Could you check a few things on this model? Use its own coordinates, in mm. A direction names the side the tool comes from. Give positions to 0.01 mm unless a question says otherwise; leave off trailing zeros. Order: outer loops, then holes, each group sorted by start corner. A loop starts at its lowest first (then second) coordinate and runs counter-clockwise, first axis right, second up.
(1) Imagine slicing it at D-D, the plane y = 68.5. Write out the boundary of the cut face in (x, z).
(2) Will these pins go through, and if not, where does the flat tip stop? pin 1 (6 mm diameter, centred on y = 62, z = 19.5, fed in from -X); pin 2 (8 mm diameter, centred on x = -64.5, y = 23.5, fed in from +Z); pin 3 (10.5 mm diameter, centred on y = 79.5, z = 12.5, fed in from +X).
(3) Imagine slicing it at A-A, the plane z = 0. Write out the boundary of the cut face in (x, y), then the cut area to 3 significant figures.
(4) On a 3-axis mill with a long thin cutter (end or side, diameter ignored), from which of +Z, -Z, +X, -X, +Y, -Y can I reach the whole of each face in a straight line? I mean faces 4 (the flat face through (-50, 49, -32)), 5 (the flat face through (-75, 63, 15)), 6 (the flat face through (0, 17, 1)), 7 (the flat face through (27, 65, 12)). Say none if no direction works.
(5) Imagine slicing it at C-C, the plane x = 61.5. Write out the boundary of the cut face in (y, z), then the cut area to 3 significant figures.
(6) Imagine slicing it at B-B, the plane x = -108.5. Write out the boundary of the cut face in (y, z), then the cut area to 3 significant figures.
(7) If I drill on probe 1 along Z at (x, y) = (50, 54); probe 2 along Z at (x, y) = (-91.5, 92); probe 3 along X at (y, z) = (50, 0), over which ranges is the centre line in solid material (lowest first)?
(8) If we mould it in two halves opening along X, with no side actions, what happens to faces 1 (the cylindrical face through (25.024, 50.21, -1.099)), 2 (the flat face through (0, 82, 1)), 3 (the cylindrical face through (-124.46, 7.61, 0.21))? For each: released by +X, released by -X, zero draft, split by the parting line, or undercut.
from build123d import *

# Parameters (mm, degrees)
BOSS_EXTRUDE1_DEPTH = 100
SKETCH4_R           = 25
CUT_EXTRUDE2_DEPTH  = 100
SKETCH6_W           = 100.520267533
SKETCH6_H           = 35
CUT_EXTRUDE4_DEPTH  = 100
BOSS_EXTRUDE3_DEPTH = 15
SKETCH11_R          = 25
CUT_EXTRUDE5_DEPTH  = 30
CUT_EXTRUDE6_DEPTH  = 30


with BuildPart() as part:
    # Sketch2 → Boss-Extrude1 (new body)
    with BuildSketch(Plane(origin=(0, 0, 0), x_dir=(1, 0, 0), z_dir=(0, 1, 0))):
        with BuildLine():
            Line((-50, 50), (50, 50))
            ThreePointArc((50, 50), (100, 0), (50, -50))
            Line((50, -50), (-50, -50))
            Line((-50, -50), (-50, 50))
        make_face()
    extrude(amount=BOSS_EXTRUDE1_DEPTH)

    # Sketch4 → Cut-Extrude2 (cut)
    with BuildSketch(Plane(origin=(0, 100, 0), x_dir=(1, 0, 0), z_dir=(0, 1, 0))):
        with Locations((50, 0)):
            Circle(SKETCH4_R)
    extrude(amount=-CUT_EXTRUDE2_DEPTH, mode=Mode.SUBTRACT)

    # Sketch6 → Cut-Extrude4 (cut)
    with BuildSketch(Plane.XY.offset(50)):
        with Locations((50.260133767, 17.5)):
            Rectangle(SKETCH6_W, SKETCH6_H)
        with Locations((50.260133767, 82.5)):
            Rectangle(SKETCH6_W, SKETCH6_H)
    extrude(amount=-CUT_EXTRUDE4_DEPTH, mode=Mode.SUBTRACT)

    # Sketch10 → Boss-Extrude3 (add, symmetric)
    with BuildSketch(Plane.XY):
        with BuildLine():
            Line((-97.564584058, 101.159083353), (-50, 100))
            Line((-50, 100), (-50, 0))
            Line((-50, 0), (-100, 1.218431082))
            ThreePointArc((-100, 1.218431082), (-149.985160866, 52.436500555), (-97.564584058, 101.159083353))
        make_face()
    extrude(amount=BOSS_EXTRUDE3_DEPTH, both=True)

    # Sketch11 → Cut-Extrude5 (cut)
    with BuildSketch(Plane.XY.offset(15)):
        with Locations((-100, 51.218431082)):
            Circle(SKETCH11_R)
    extrude(amount=-CUT_EXTRUDE5_DEPTH, mode=Mode.SUBTRACT)

    # Sketch12 → Cut-Extrude6 (cut)
    with BuildSketch(Plane.XY.offset(15)):
        Polygon((-218.838630954, 25.001308264), (-99.744243338, 26.219739346), (-100.255756662, 76.217122818), (-219.350144278, 74.998691736), align=None)
    extrude(amount=-CUT_EXTRUDE6_DEPTH, mode=Mode.SUBTRACT)


solid = part.part
Answer block:
1. outline: (-81.93, -15) - (-50, -15) - (-50, -50) - (0, -50) - (0, 50) - (-50, 50) - (-50, 15) - (-81.93, 15) - close
2. pin 1: stops at x = -50
2. pin 2: stops at z = 15
2. pin 3: stops at x = 0
3. outline: (-143.55, 75.77) - (-100.26, 76.22) arc R25 cw to (-99.74, 26.22) - (-143.04, 25.78) arc R50 ccw to (-100, 1.22) - (-50, 0) - (0, 0) - (0, 35) - (25, 35) - (25, 65) - (0, 65) - (0, 100) - (-50, 100) - (-97.56, 101.16) arc R50 ccw to start; (75, 35) - (100, 35) - (100, 65) - (75, 65) - close
3. area: 12,100 mm2
4. face 4: -Z, -X, +Y, -Y
4. face 5: +Z, -X, +Y, -Y
4. face 6: +Z, -Z, +X, -Y
4. face 7: +Z, -Z, +X, +Y
5. outline: (35, -48.66) - (65, -48.66) - (65, -22.2) - (35, -22.2) - close; (35, 22.2) - (65, 22.2) - (65, 48.66) - (35, 48.66) - close
5. area: 1,590 mm2
6. outline: (1.95, -15) - (26.13, -15) - (26.13, 15) - (1.95, 15) - close; (76.13, -15) - (100.49, -15) - (100.49, 15) - (76.13, 15) - close
6. area: 1,460 mm2
7. probe 1: z = -50 to -25, 25 to 50
7. probe 2: z = -15 to 15
7. probe 3: x = -75.03 to 25, 75 to 100
8. face 1: undercut
8. face 2: released by +X
8. face 3: released by -X
